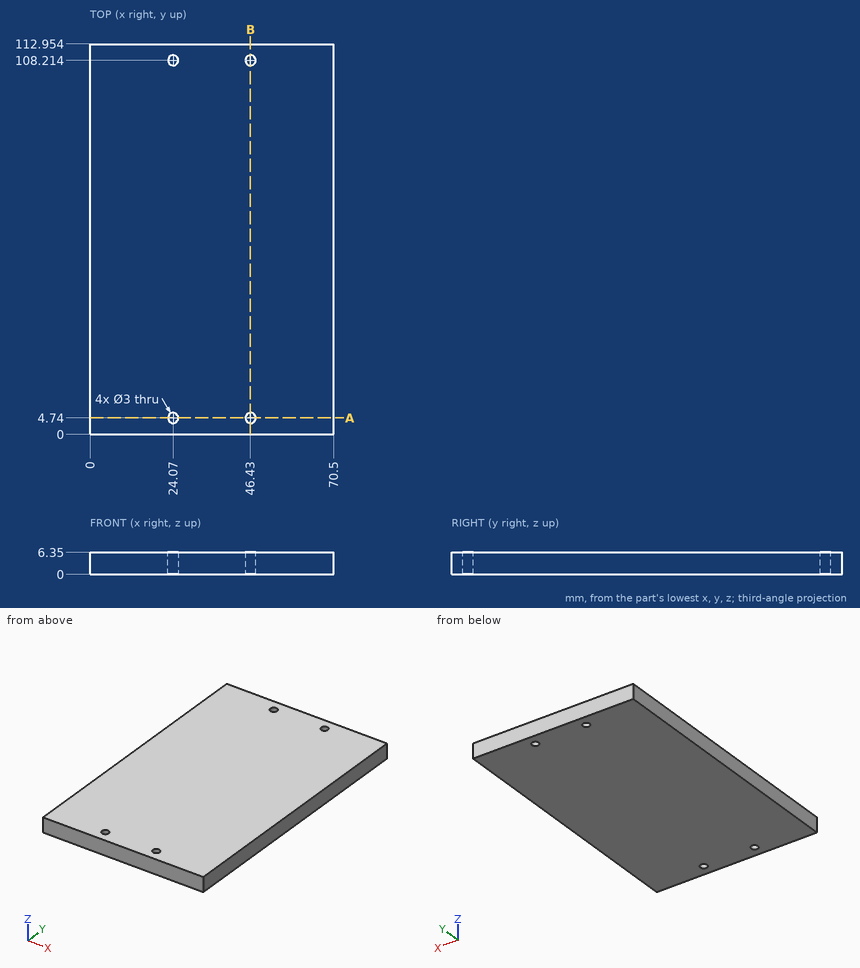
Geometry: see drawing. Coordinates: mm, zero at the bounding-box minimum. Coordinates: 2 decimals unless noted, no trailing zeros. Write each loop counter-clockwise with the first axis right and the second up, starting at its lowest first coordinate (ties: lowest second). Pieces come first, ordered by that corner, then holes.
1) Section A-A on y = 4.74. Output: boundary loops of the cut face in (x, z), and give its area (3 significant figures).
2) Material intervals for line 1 along Y through (x, z) = (46.43, 4); line 2 along X through (y, z) = (107.5, 1.75); line 3 along X through (y, z) = (6, 5.5) (1 decimal), sorted ascending.
3) Section B-B on x = 46.43. Output: boundary loops of the cut face in (y, z).
Check result:
1. outline: (0, 0) - (22.57, 0) - (22.57, 6.35) - (0, 6.35) - close; (25.57, 0) - (44.93, 0) - (44.93, 6.35) - (25.57, 6.35) - close; (47.93, 0) - (70.5, 0) - (70.5, 6.35) - (47.93, 6.35) - close
1. area: 410 mm2
2. line 1: y = 0 to 3.24, 6.24 to 106.71, 109.71 to 112.95
2. line 2: x = 0 to 22.75, 25.39 to 45.11, 47.75 to 70.5
2. line 3: x = 0 to 23.3, 24.9 to 45.6, 47.2 to 70.5
3. outline: (0, 0) - (3.24, 0) - (3.24, 6.35) - (0, 6.35) - close; (6.24, 0) - (106.71, 0) - (106.71, 6.35) - (6.24, 6.35) - close; (109.71, 0) - (112.95, 0) - (112.95, 6.35) - (109.71, 6.35) - close
